```python
from build123d import *

# Parameters (mm, degrees)
SKETCH1_W                  = 200
SKETCH1_H                  = 200
BOSS_EXTRUDE1_DEPTH        = 10
SKETCH2_R                  = 32.5
SKETCH2_R_2                = 25
BOSS_EXTRUDE2_DEPTH        = 75
RIB1_REACH                 = 167
SKETCH3_WALL_W             = 401.282032302
SKETCH3_WALL_H             = 10
CIRPATTERN1_COUNT          = 4
MOUNTING_HOLES_D           = 11
MOUNTING_HOLES_CSINK_D     = 13.5
MOUNTING_HOLES_CSINK_ANGLE = 90
FILLET1_R                  = 20
FILLET2_R                  = 40
CHAMFER1_SIZE              = 2.5
CHAMFER2_SIZE              = 1


# Read off the part's stored shape, not the designer's step: M6x1.0 Tapped Hole1, M6x1.0 Tapped Hole2
with BuildPart() as part:
    # Sketch1 → Boss-Extrude1 (new body)
    with BuildSketch(Plane(origin=(0, 0, 0), x_dir=(1, 0, 0), z_dir=(0, 1, 0))):
        Rectangle(SKETCH1_W, SKETCH1_H)
    extrude(amount=BOSS_EXTRUDE1_DEPTH)

    # Sketch2 → Boss-Extrude2 (add)
    with BuildSketch(Plane(origin=(0, 10, 0), x_dir=(1, 0, 0), z_dir=(0, 1, 0))):
        with Locations(Location((0, 0, 0), (0, 0, 90))):
            Circle(SKETCH2_R)
        with Locations(Location((0, 0, 0), (0, 0, 270))):
            Circle(SKETCH2_R_2, mode=Mode.SUBTRACT)
    extrude(amount=BOSS_EXTRUDE2_DEPTH)

    # Sketch3 wall → Rib1 (add, up to next)
    with BuildSketch(Plane(origin=(49.820508076, 40, 0), x_dir=(0.499999999996, -0.866025403787, 0), z_dir=(0.866025403787, 0.499999999996, 0)), mode=Mode.PRIVATE) as rib1_sk1:
        Rectangle(SKETCH3_WALL_W, SKETCH3_WALL_H)
    rib1_tool1 = extrude(rib1_sk1.sketch, amount=-RIB1_REACH, mode=Mode.PRIVATE) - part.part
    rib1 = rib1_tool1.solids().sort_by_distance((49.820508076, 40, 0))[0]
    add(rib1)

    # CirPattern1: Rib1 ×4 about axis
    cirpattern1_axis = Axis((0, 0, 0), (0, 1, 0))
    for i in range(1, CIRPATTERN1_COUNT):
        add(rib1.rotate(cirpattern1_axis, i * 360 / CIRPATTERN1_COUNT))

    # M6x1.0 Tapped Hole1 outline → M6x1.0 Tapped Hole1 (revolve, cut)
    with BuildSketch(Plane(origin=(0, 60, 0), x_dir=(0.707106781186546, 0, 0.707106781186549), z_dir=(0, 1, 0))):
        Polygon((0, -32.500112934), (3.750112934, -32.500112934), (2.5, -31.25), (2.5, -24.874618187), (0, -24.874618187), align=None)
    revolve(axis=Axis((0, 60, 0), (0.707106781186549, 0, -0.707106781186546)), mode=Mode.SUBTRACT)

    # M6x1.0 Tapped Hole2 outline → M6x1.0 Tapped Hole2 (revolve, cut)
    with BuildSketch(Plane(origin=(0, 60, 0), x_dir=(0.707106781186546, 0, -0.707106781186549), z_dir=(0, -1, 0))):
        Polygon((3.750104401, 32.500104401), (0, 32.500104401), (0, 24.874618187), (2.5, 24.874618187), (2.5, 31.25), align=None)
    revolve(axis=Axis((0, 60, 0), (0.707106781186549, 0, 0.707106781186546)), mode=Mode.SUBTRACT)

    # Mounting Holes (through all)
    with Locations(Plane(origin=(0, 10, 0), x_dir=(1, 0, 0), z_dir=(0, 1, 0))):
        with Locations((-62.5, 62.5), (62.5, 62.5), (62.5, -62.5), (-62.5, -62.5)):
            CounterSinkHole(MOUNTING_HOLES_D / 2, MOUNTING_HOLES_CSINK_D / 2, counter_sink_angle=MOUNTING_HOLES_CSINK_ANGLE)

    # Fillet1
    fillet1_edges = [part.edges().sort_by_distance(p)[0] for p in [
        (-22.980970389, 10, -22.980970389),
        (22.980970389, 10, -22.980970389),
        (22.980970389, 10, 22.980970389),
        (-22.980970389, 10, 22.980970389),
    ]]
    fillet(fillet1_edges, radius=FILLET1_R)

    # Fillet2
    fillet2_edges = [part.edges().sort_by_distance(p)[0] for p in [
        (100, 5, 100),
        (-100, 5, 100),
        (-100, 5, -100),
        (100, 5, -100),
    ]]
    fillet(fillet2_edges, radius=FILLET2_R)

    # Chamfer1
    chamfer1_edges = [part.edges().sort_by_distance(p)[0] for p in [
        (-100, 10, 0),
        (0, 10, -100),
        (0, 10, 100),
        (100, 10, 0),
        (-88.284271247, 10, 88.284271247),
        (88.284271247, 10, 88.284271247),
        (88.284271247, 10, -88.284271247),
        (-88.284271247, 10, -88.284271247),
    ]]
    chamfer(chamfer1_edges, length=CHAMFER1_SIZE)

    # Chamfer2
    chamfer2_edges = [part.edges().sort_by_distance(p)[0] for p in [
        (-49.627048799, 40.335081297, -5),
        (-49.627048799, 40.335081297, 5),
        (-5, 40.335081297, 49.627048799),
        (5, 40.335081297, 49.627048799),
        (49.627048799, 40.335081297, 5),
        (49.627048799, 40.335081297, -5),
        (-5, 40.335081297, -49.627048799),
        (5, 40.335081297, -49.627048799),
    ]]
    chamfer(chamfer2_edges, length=CHAMFER2_SIZE)


solid = part.part
```
Source: CAD feature listing. Evaluate the final solid. Frame: model axes, mm. A direction names the side the tool comes from. Coordinates: 2 decimals unless noted, no trailing zeros. Order: outer loops, then holes, each group sorted by start corner. A loop starts at its lowest first (then second) coordinate and runs counter-clockwise, first axis right, second up. Notation, with made-up numbers: (41, 18.25) - (69, 18.25) arc R13 ccw to (69, 42.25) - close; hole circle Ø3 at (54.5, 71.5). An arc over 180 degrees is marked (long way). One line per item, written item: value.
1) Contact query for flat-ended pins moving along their axis: pin 1 (1.5 mm diameter, centred on x = 3.5, y = 15, fed in from -Z); pin 2 (10 mm diameter, centred on y = 37, z = -18.5, fed in from +X); pin 3 (12 mm diameter, centred on x = -20, z = 74, fed in from +Y); pin 4 (2 mm diameter, centred on x = -51, z = 15.5, fed in from -Y). Output: stop coordinate, or through.
Computed values:
pin 1: stops at z = -64.69
pin 2: stops at x = 29.56
pin 3: stops at y = 10
pin 4: stops at y = 0
2) Ray query, line 1 (Z direction, x = 62, y = 3); line 2 (Y direction, x = 73.5, z = 40). Return the intervals inside material, ascending. Write a range as [from, to].
Computed values:
line 1: z = [-99.95, -67.98], [-57.02, 57.02], [67.98, 99.95]
line 2: y = [0, 10]
3) Cut plane B-B on z = 0. Output: boundary loops of the cut face in (x, y).
Computed values:
outline: (-100, 0) - (100, 0) - (100, 7.5) - (97.5, 10) - (67.14, 10) - (32.5, 70) - (32.5, 85) - (25, 85) - (25, 10) - (-25, 10) - (-25, 85) - (-32.5, 85) - (-32.5, 70) - (-67.14, 10) - (-97.5, 10) - (-100, 7.5) - close
4) Mould query, pull axis X, two halves, no side actions, for faces 5 (the face through (-18.86, 57.89, 20.76)), 6 (the face through (49.45, 40.64, -0.06)), 7 (the face through (-86.918, 9.844, -86.333)). Classes: released by +X, released by -X, zero draft, split by the parting line, or undercut.
Computed values:
face 5: undercut
face 6: released by +X
face 7: released by -X
5) Cut plane D-D on x = 62.5. State how many separate pieces and enclosed holes the cut face has, plus the area to 3 significant figures.
Computed values:
separate pieces: 3
enclosed holes: 0
area: 1,850 mm^2
6) Reachability of faces 1 (the face through (5, 29, 45)), 2 (the face through (49.03, 40.39, -4.49)), 3 (the face through (-5, 29, 45)), 4 (the face through (0, 10, 0)) from +Z, -Z, +X, -X, +Y, -Y: full face, straight path, thin tool, end or side. Return the list, or none.
Computed values:
face 1: +Z, +X, +Y
face 2: -Z, +X, +Y
face 3: +Z, -X, +Y
face 4: +Y
7) Cut plane C-C on y = 45.5. Output: boundary loops of the cut face in (x, z), plus the area to 3 significant figures.
Computed values:
outline: (-46.65, -4) - (-45.49, -5) - (-32.11, -5) arc R32.5 ccw to (-5, -32.11) - (-5, -45.49) - (-4, -46.65) - (4, -46.65) - (5, -45.49) - (5, -32.11) arc R32.5 ccw to (32.11, -5) - (45.49, -5) - (46.65, -4) - (46.65, 4) - (45.49, 5) - (32.11, 5) arc R32.5 ccw to (5, 32.11) - (5, 45.49) - (4, 46.65) - (-4, 46.65) - (-5, 45.49) - (-5, 32.11) arc R32.5 ccw to (-32.11, 5) - (-45.49, 5) - (-46.65, 4) - close; hole circle Ø50 at (0, 0)
area: 1,920 mm^2
8) Cut plane A-A on x = 0. Output: boundary loops of the cut face in (y, z).
Computed values:
outline: (0, -100) - (7.5, -100) - (10, -97.5) - (10, -67.14) - (70, -32.5) - (85, -32.5) - (85, -25) - (10, -25) - (10, 25) - (85, 25) - (85, 32.5) - (70, 32.5) - (10, 67.14) - (10, 97.5) - (7.5, 100) - (0, 100) - close
